Check sheet for the modelled part. Datum: model origin and axes. Units: mm. Face numbers are marked on the shaded views. A direction names the side the tool comes from. Coordinates: 2 decimals unless noted, no trailing zeros. Write each loop counter-clockwise with the first axis right and the second up, starting at its lowest first coordinate (ties: lowest second). Pieces come first, ordered by that corner, then holes. Notation, with made-up numbers: M 89,21.25 L 128,21.25 A8 ccw 128,31.25 Z; hole C -39.75,51 d4. An arc over 180 degrees is marked long. Answer as CSV lines item,"result".
from build123d import *

# Parameters (mm, degrees)
BOSS_EXTRUDE1_DEPTH    = 36
SKETCH2_R              = 10.5
CUT_EXTRUDE1_DEPTH     = 74.491730036
SKETCH3_W              = 18.5
SKETCH3_H              = 29
CUT_EXTRUDE2_DEPTH     = 78.024618067
RIB1_REACH             = 75.682
SKETCH4_WALL_W         = 186.1063102
SKETCH4_WALL_H         = 2
RIB2_REACH             = 75.682
SKETCH5_WALL_W         = 186.1063102
SKETCH5_WALL_H         = 2
CHAMFER1_SIZE          = 3
BOSS_EXTRUDE2_START    = -2
SKETCH6_R              = 10.5
SKETCH6_R_2            = 9
BOSS_EXTRUDE2_DEPTH    = 2
M2_5_CLEARANCE_HOLE1_D = 2.9
SKETCH10_R             = 15
SKETCH10_R_2           = 11
CUT_EXTRUDE4_DEPTH     = 0.6


with BuildPart() as part:
    # Sketch1 → Boss-Extrude1 (new body)
    with BuildSketch(Plane.XY):
        Polygon((0, 0), (17, 0), (17, 29), (0.843441467, 29), (0.843441467, 62), (-11.156558533, 62), (-11.156558533, 25), (0, 25), align=None)
    extrude(amount=BOSS_EXTRUDE1_DEPTH)

    # Sketch2 → Cut-Extrude1 (cut, through all)
    with BuildSketch(Plane(origin=(0.843441467, 0, 0), x_dir=(0, 0, -1), z_dir=(1, 0, 0))):
        with Locations(Location((-18, 45, 0), (0, 0, 90))):
            Circle(SKETCH2_R)
    extrude(amount=-CUT_EXTRUDE1_DEPTH, mode=Mode.SUBTRACT)

    # Sketch3 → Cut-Extrude2 (cut, through all)
    with BuildSketch(Plane(origin=(17, 0, 0), x_dir=(0, 0, -1), z_dir=(1, 0, 0))):
        with Locations((-18, 14.5)):
            Rectangle(SKETCH3_W, SKETCH3_H)
    extrude(amount=-CUT_EXTRUDE2_DEPTH, mode=Mode.SUBTRACT)

    # Sketch4 wall → Rib1 (add, up to next)
    with BuildSketch(Plane(origin=(8.921720734, 45.5, 36), x_dir=(0.439720227065, -0.898134801636, 0), z_dir=(0.898134801636, 0.439720227065, 0)), mode=Mode.PRIVATE) as rib1_sk1:
        with Locations((0, 1)):
            Rectangle(SKETCH4_WALL_W, SKETCH4_WALL_H)
    rib1_tool1 = extrude(rib1_sk1.sketch, amount=-RIB1_REACH, mode=Mode.PRIVATE) - part.part
    add(rib1_tool1.solids().sort_by_distance((8.921720734, 45.5, 36))[0])

    # Sketch5 wall → Rib2 (add, up to next)
    with BuildSketch(Plane(origin=(8.921720734, 45.5, 0), x_dir=(0.439720227065, -0.898134801636, 0), z_dir=(-0.898134801636, -0.439720227065, 0)), mode=Mode.PRIVATE) as rib2_sk1:
        with Locations((0, 1)):
            Rectangle(SKETCH5_WALL_W, SKETCH5_WALL_H)
    rib2_tool1 = extrude(rib2_sk1.sketch, amount=RIB2_REACH, mode=Mode.PRIVATE) - part.part
    add(rib2_tool1.solids().sort_by_distance((8.921720734, 45.5, 0))[0])

    # Chamfer1
    chamfer1_edges = [part.edges().sort_by_distance(p)[0] for p in [
        (8.921720733, 29, 8.75),
        (8.921720733, 29, 27.25),
    ]]
    chamfer(chamfer1_edges, length=CHAMFER1_SIZE)

    # Sketch6 → Boss-Extrude2 (add)
    with BuildSketch(Plane.ZY.offset(11.156558533).offset(BOSS_EXTRUDE2_START)):
        with Locations(Location((18, 45, 0), (0, 0, 90))):
            Circle(SKETCH6_R)
        with Locations(Location((18, 45, 0), (0, 0, 270))):
            Circle(SKETCH6_R_2, mode=Mode.SUBTRACT)
    extrude(amount=BOSS_EXTRUDE2_DEPTH)

    # M2.5 Clearance Hole1 (through all)
    with Locations(Plane.XY.offset(36)):
        with Locations((2.5, 9.75), (14.5, 9.75)):
            Hole(M2_5_CLEARANCE_HOLE1_D / 2)

    # Sketch10 → Cut-Extrude4 (cut)
    with BuildSketch(Plane.ZY.offset(11.156558533)):
        with Locations(Location((18, 45, 0), (0, 0, 270))):
            Circle(SKETCH10_R)
        with Locations(Location((18, 45, 0), (0, 0, 270))):
            Circle(SKETCH10_R_2, mode=Mode.SUBTRACT)
    extrude(amount=-CUT_EXTRUDE4_DEPTH, mode=Mode.SUBTRACT)


solid = part.part
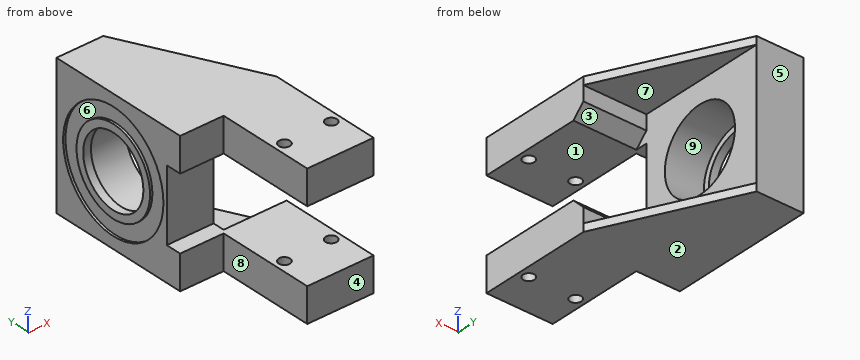
1) Section check B-B, the plane x = -3. Record the boundary of the cut face in (y, z).
Answer key:
outline,"M 25,0 L 62,0 L 62,36 L 25,36 L 25,27.25 L 29,27.25 L 29,8.75 L 25,8.75 Z; hole C 45,18 d21"
2) Depth check by flat-ended pin: P1, Ø1, axis at x = -3.5, z = 23.5, coming from the -Y side; P2, Ø9.5, axis at y = 6.5, z = 5, coming from the -X side; P3, Ø2.5, axis at x = -6.5, z = 33, coming from the -Y side. Enter the tip coordinate at first touch or a pass-through.
Answer key:
P1,"stops at y = 29"
P2,"stops at x = 0"
P3,"stops at y = 25"
3) Section check D-D, the plane y = 17.5. Record the boundary of the cut face in (x, z).
Answer key:
outline,"M 0,0 L 17,0 L 17,8.75 L 0,8.75 Z; M 0,27.25 L 17,27.25 L 17,36 L 0,36 Z"
4) Section check A-A, the plane y = 9.75. Record the boundary of the cut face in (x, z), plus the area to 3 significant figures.
Answer key:
outline,"M 0,0 L 1.05,0 L 1.05,8.75 L 0,8.75 Z; M 0,27.25 L 1.05,27.25 L 1.05,36 L 0,36 Z; M 3.95,0 L 13.05,0 L 13.05,8.75 L 3.95,8.75 Z; M 3.95,27.25 L 13.05,27.25 L 13.05,36 L 3.95,36 Z; M 15.95,0 L 17,0 L 17,8.75 L 15.95,8.75 Z; M 15.95,27.25 L 17,27.25 L 17,36 L 15.95,36 Z"
area,"196 mm2"
5) Section check C-C, the plane z = 18. Record the boundary of the cut face in (x, y), plus the area to 3 significant figures.
Answer key:
outline,"M -11.16,29 L 0.84,29 L 0.84,34.5 L -9.16,34.5 L -9.16,36 L -11.16,36 L -11.16,34 L -10.56,34 L -10.56,30 L -11.16,30 Z; M -11.16,54 L -9.16,54 L -9.16,55.5 L 0.84,55.5 L 0.84,62 L -11.16,62 L -11.16,60 L -10.56,60 L -10.56,56 L -11.16,56 Z"
area,"145 mm2"
6) Mould release check, pull along Z, two halves, no side actions. Record for the marked faces 1, 2, 3 and 4: pulls with the +Z half, pulls with the -Z half, needs draft (parallel to the pull), parting line crosses it, or undercut.
Answer key:
face 1,"undercut"
face 2,"pulls with the -Z half"
face 3,"undercut"
face 4,"needs draft"
7) Thickness scan on line 1 along Z through (x, y) = (-9.65, 45); line 2 along Y through (x, z) = (2.5, 2.25); line 3 along Z through (x, y) = (5, 10). Record the ranges inside material, lowest first.
Answer key:
line 1,"z = 0 to 9, 27 to 36"
line 2,"y = 0 to 8.3, 11.2 to 29"
line 3,"z = 0 to 8.75, 27.25 to 36"
8) Tool access check on the marked faces 5, 6, 7, 8 and 9. Record the directions out of +Z, -Z, +X, -X, +Y, -Y that give a thin tool (end or side, any length) a straight path to the whole face; none if there is none.
Answer key:
face 5,"+Z, -Z, +X, -X, +Y"
face 6,"-X"
face 7,"+X, +Y"
face 8,"+Z, -Z, -X, -Y"
face 9,"+X"
